Check sheet for the drawn part. Datum: minimum x, y, z corner. Units: mm. A direction names the side the tool comes from. Round coordinates to 2 decimals unless told otherwise and drop trailing zeros. Write each loop counter-clockwise with the first axis right and the second up, starting at its lowest first coordinate (ties: lowest second). Pieces come first, ordered by that corner, then holes. Notation, with made-up numbers: M 30.5,67.5 L 88.5,67.5 A13 cw 88.5,83.5 Z; hole C 25,-7 d1. An arc over 180 degrees is marked long. Put each result on its own line as item: value.
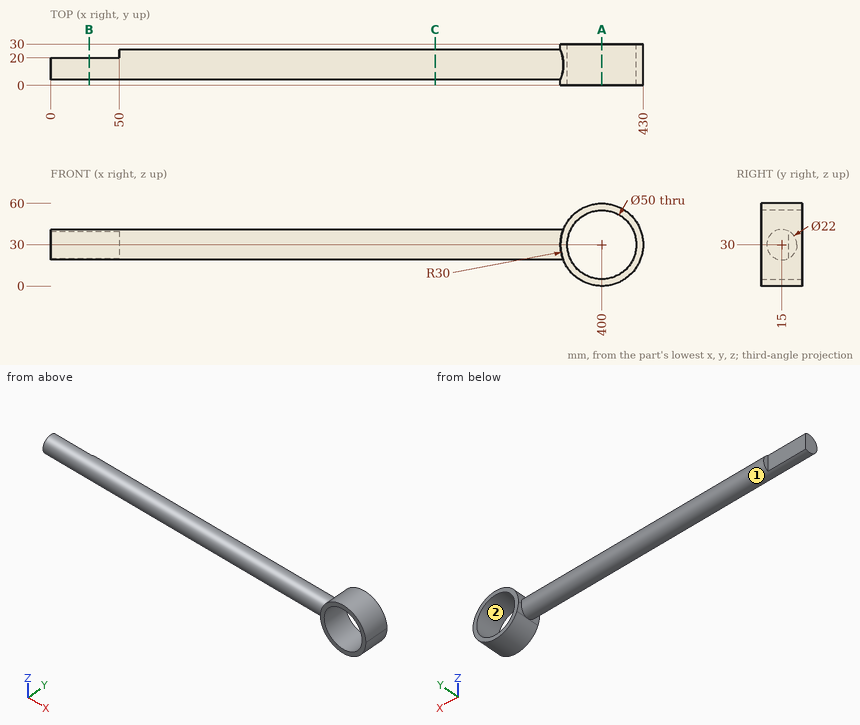
1. Depth check by flat-ended pin: pin 1 Ø21.5 at (x, z) = (32, 30.5) entering from +Y; pin 2 Ø1.5 at (x, y) = (243, 18.5) entering from -Z; pin 3 Ø2 at (x, z) = (53.5, 25) entering from +Y. Enter the tip coordinate at first touch or a pass-through.
Computed values:
pin 1: stops at y = 20
pin 2: stops at z = 19.35
pin 3: stops at y = 25.25
2. Cross-section at A-A (x = 400). Enter the section's corners in (y, z).
Computed values:
outline: M 0,0 L 30,0 L 30,5 L 0,5 Z; M 0,55 L 30,55 L 30,60 L 0,60 Z
3. Scan lines: probe 1 along X at (y, z) = (21, 30); probe 2 along Y at (x, z) = (365, 30); probe 3 along X at (y, z) = (25, 22.5). Record each from-to range of solid material in increasing order.
Computed values:
probe 1: x = 50 to 375, 425 to 430
probe 2: y = 4 to 26
probe 3: x = 370.95 to 376.15, 423.85 to 429.05
4. Cross-section at C-C (x = 279). Enter the section's corners in (y, z).
Computed values:
outline: C 15,30 d22
5. Cross-section at B-B (x = 28). Enter the section's corners in (y, z), then the cut area to 3 significant figures.
Computed values:
outline: M 20,20.2 L 20,39.8 A11 ccw long Z
area: 296 mm2
6. Access from +Z, -Z, +X, -X, +Y, -Y to the whole of each face (thin tool, end or side, straight path). Record for the marked faces 1 and 2.
Computed values:
face 1: -X
face 2: +Y, -Y
